Geometry check sheet. Reference: drawing and pictorial views, mm from the part's lowest x, y, z. A direction names the side the tool comes from. Round coordinates to 2 decimals unless told otherwise and drop trailing zeros. Write each loop counter-clockwise with the first axis right and the second up, starting at its lowest first coordinate (ties: lowest second). Pieces come first, ordered by that corner, then holes. Notation, with made-up numbers: M 46.5,55 L 65.5,55 A15 ccw 65.5,80 Z; hole C -6.5,50 d1. An arc over 180 degrees is marked long. Put each result on its own line as item: value. Start each with the question number.
(1) Mould release check, pull along X, two halves, no side actions. Record for the marked faces 1, 2 and 3: pulls with the +X half, pulls with the -X half, needs draft (parallel to the pull), parting line crosses it, or undercut.
(2) Section check C-C on y = 41. Record the cut outline in (x, z), then the cut area to 3 significant figures.
(3) Material ranges on probe 1 along Y at (x, z) = (8.75, 6.5); probe 2 along Y at (x, z) = (17.75, 9.5); probe 3 along Y at (x, z) = (17, 4.5), recorded low to high.
(4) Section check D-D on y = 23.5. Record the cut outline in (x, z), then the cut area to 3 significant figures.
(5) Section check B-B on x = 10.5. Record the cut outline in (y, z).
(6) Section check A-A on z = 7.25. Record the cut outline in (x, y), then the cut area to 3 significant figures.
(7) Tool access check on the marked faces 4 and 5. Record the directions out of +Z, -Z, +X, -X, +Y, -Y that give a thin tool (end or side, any length) a straight path to the whole face; none if there is none.
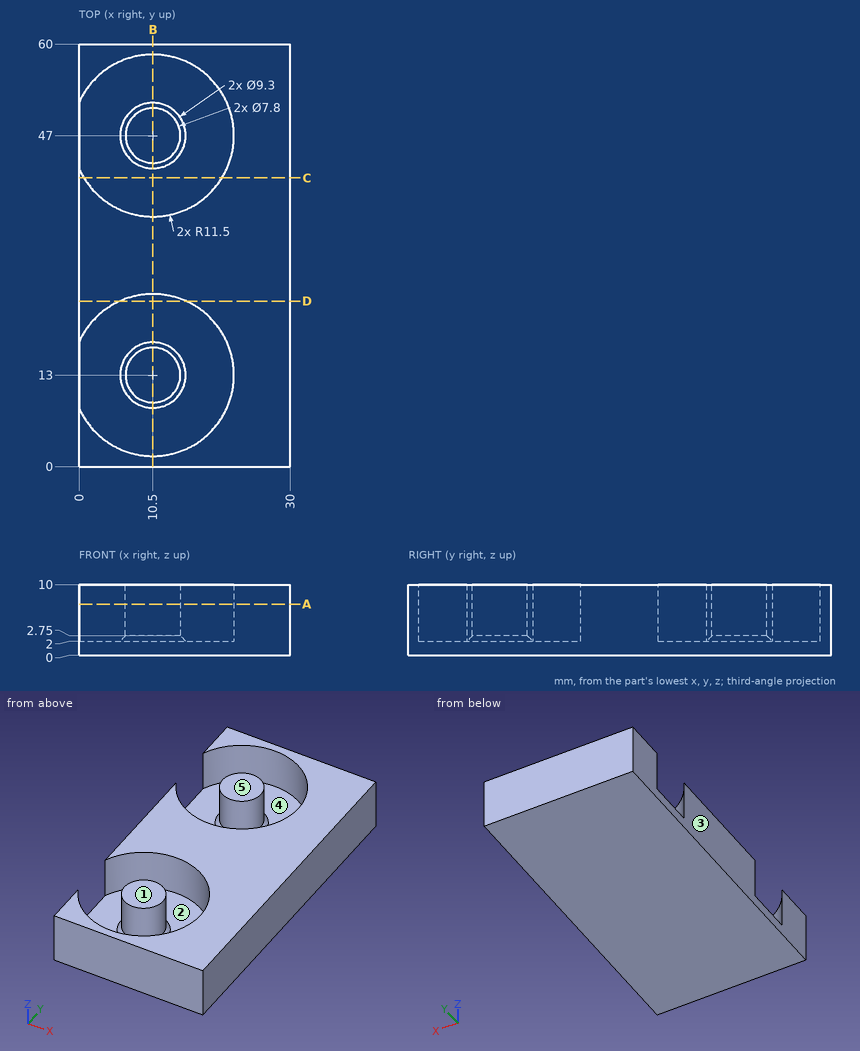
Answers follow:
1. face 1: needs draft
1. face 2: undercut
1. face 3: pulls with the -X half
2. outline: M 0,0 L 30,0 L 30,10 L 20.31,10 L 20.31,2 L 0.69,2 L 0.69,10 L 0,10 Z
2. area: 143 mm^2
3. probe 1: y = 0 to 1.63, 9.51 to 16.49, 24.37 to 35.63, 43.51 to 50.49, 58.37 to 60
3. probe 2: y = 0 to 4.07, 21.93 to 38.07, 55.93 to 60
3. probe 3: y = 0 to 3.51, 22.49 to 37.51, 56.49 to 60
4. outline: M 0,0 L 30,0 L 30,10 L 15.19,10 L 15.19,2 L 5.81,2 L 5.81,10 L 0,10 Z
4. area: 225 mm^2
5. outline: M 0,0 L 60,0 L 60,10 L 58.5,10 L 58.5,2 L 51.65,2 L 50.9,2.75 L 50.9,10 L 43.1,10 L 43.1,2.75 L 42.35,2 L 35.5,2 L 35.5,10 L 24.5,10 L 24.5,2 L 17.65,2 L 16.9,2.75 L 16.9,10 L 9.1,10 L 9.1,2.75 L 8.35,2 L 1.5,2 L 1.5,10 L 0,10 Z
6. outline: M 0,0 L 30,0 L 30,60 L 0,60 L 0,51.69 A11.5 cw long 0,42.31 L 0,17.69 A11.5 cw long 0,8.31 Z; C 10.5,13 d7.8; C 10.5,47 d7.8
6. area: 1,080 mm^2
7. face 4: +Z
7. face 5: +Z, +X, -X, +Y, -Y
